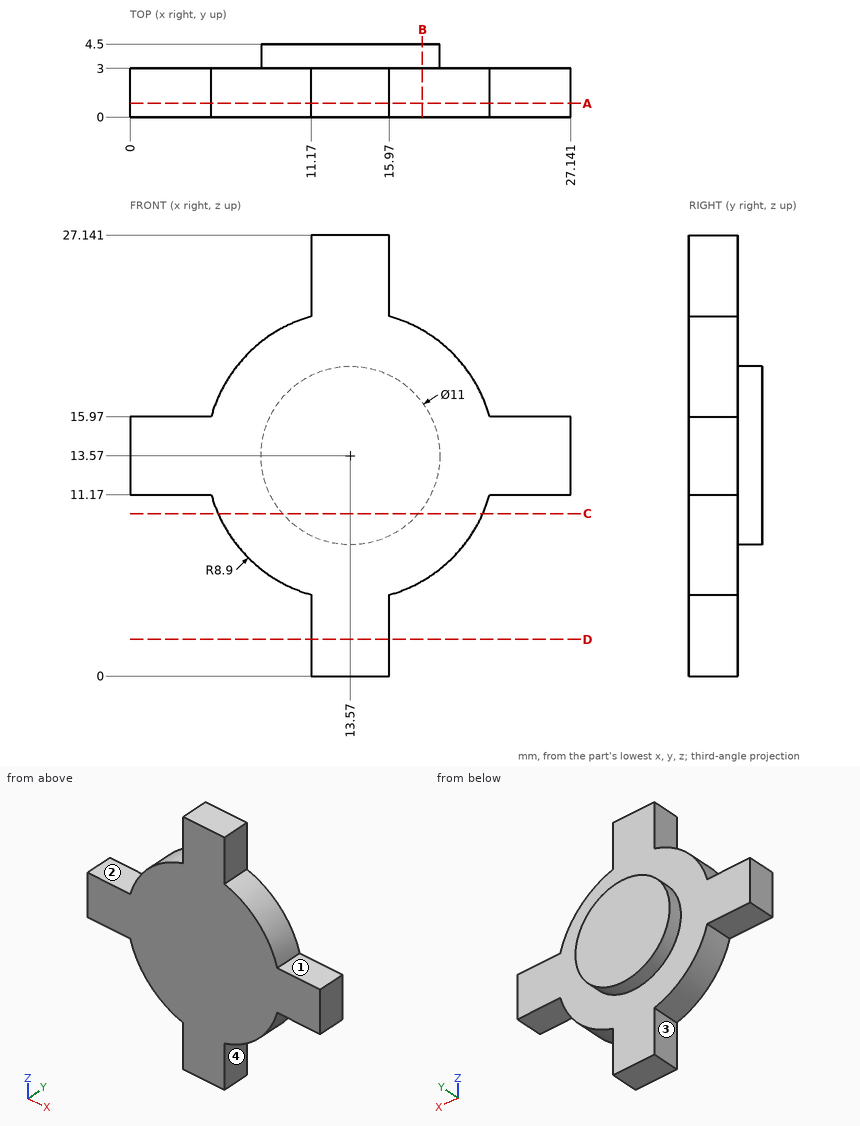
Input: dimensioned drawing with shaded views. Units: mm. Origin: part minimum x, y, z. A direction names the side the tool comes from. Coordinates: 2 decimals unless noted, no trailing zeros. Loops run counter-clockwise (first coordinate to the right, second up) from the corner with the lowest first, then second, coordinate; pieces in that order, holes last.
Q1. Contact query for flat-ended pins moving along their axis: pin 1 (2.5 mm diameter, centred on x = 2.5, y = 2, fed in from +Z); pin 2 (1.5 mm diameter, centred on y = 2, z = 3.5, fed in from -X); pin 3 (1 mm diameter, centred on y = 1, z = 21, fed in from -X) (1 decimal). Output: stop coordinate, or through.
Results are:
pin 1: stops at z = 15.97
pin 2: stops at x = 11.17
pin 3: stops at x = 8
Q2. Section C-C, the plane z = 10. Return the cut outline in (x, y).
Results are:
outline: (5.42, 0) - (21.72, 0) - (21.72, 3) - (17.75, 3) - (17.75, 4.5) - (9.39, 4.5) - (9.39, 3) - (5.42, 3) - close
Q3. Section B-B, the plane x = 18. Return the cut outline in (y, z).
Results are:
outline: (0, 5.85) - (3, 5.85) - (3, 10.31) - (4.5, 10.31) - (4.5, 16.83) - (3, 16.83) - (3, 21.29) - (0, 21.29) - close
Q4. Line query: line 1 along Y through (x, z) = (15, 1.5); line 2 along X through (y, z) = (1.8, 1.75). Output: solid intervals per line, ascending.
Results are:
line 1: y = 0 to 3
line 2: x = 11.17 to 15.97
Q5. Set-up query: the marked faces 1, 2, 3 and 4. Return all of +Z, -Z, +X, -X, +Y, -Y with unobstructed straight access to the full face (end or side cutting, diameter ignored); none if empty.
Results are:
face 1: +Z, +X, +Y, -Y
face 2: +Z, -X, +Y, -Y
face 3: -Z, -X, +Y, -Y
face 4: -Z, +X, +Y, -Y
Q6. Section A-A, the plane y = 0.85. Return the cut outline in (x, z), and give its area (3 significant figures).
Results are:
outline: (0, 11.17) - (5, 11.17) arc R8.9 ccw to (11.17, 5) - (11.17, 0) - (15.97, 0) - (15.97, 5) arc R8.9 ccw to (22.14, 11.17) - (27.14, 11.17) - (27.14, 15.97) - (22.14, 15.97) arc R8.9 ccw to (15.97, 22.14) - (15.97, 27.14) - (11.17, 27.14) - (11.17, 22.14) arc R8.9 ccw to (5, 15.97) - (0, 15.97) - close
area: 341 mm2
Q7. Section D-D, the plane z = 2.25. Return the cut outline in (x, y).
Results are:
outline: (11.17, 0) - (15.97, 0) - (15.97, 3) - (11.17, 3) - close
